```python
from build123d import *

# Parameters (mm, degrees)
SKETCH1_W           = 8
SKETCH1_H           = 8
SKETCH1_R           = 2.5
BOSS_EXTRUDE1_DEPTH = 2
SKETCH5_OUTSIDE_W   = 39.864
SKETCH5_OUTSIDE_H   = 39.864
SKETCH5_OUTSIDE_R   = 4
CUT_EXTRUDE2_DEPTH  = 7.92820323
CUT_EXTRUDE2_DRAFT  = -60


with BuildPart() as part:
    # Sketch1 → Boss-Extrude1 (new, symmetric)
    with BuildSketch(Plane(origin=(0, 0, 0), x_dir=(1, 0, 0), z_dir=(0, 1, 0))):
        Rectangle(SKETCH1_W, SKETCH1_H)
        with Locations(Location((0, 0, 0), (0, 0, 270))):
            Circle(SKETCH1_R, mode=Mode.SUBTRACT)
    extrude(amount=BOSS_EXTRUDE1_DEPTH, both=True)


with BuildPart() as cut_extrude2_tool:
    # Sketch5 outside → Cut-Extrude2 (with draft: the straight prism first)
    with BuildSketch(Plane(origin=(0, 2, 0), x_dir=(1, 0, 0), z_dir=(0, 1, 0))):
        Rectangle(SKETCH5_OUTSIDE_W, SKETCH5_OUTSIDE_H)
        Circle(SKETCH5_OUTSIDE_R, mode=Mode.SUBTRACT)
    extrude(amount=-CUT_EXTRUDE2_DEPTH)
    # Cut-Extrude2: the draft: its side faces are tilted about the plane it starts from
    cut_extrude2_sides = [cut_extrude2_tool.faces().sort_by_distance(p)[0] for p in [
        (0, -1.964101615, 19.932),
        (19.932, -1.964101615, 0),
        (0, -1.964101615, -19.932),
        (-19.932, -1.964101615, 0),
        (-4, -1.964101615, 0),
    ]]
    draft(cut_extrude2_sides, Plane(origin=(0, 2, 0), x_dir=(1, 0, 0), z_dir=(0, 1, 0)), CUT_EXTRUDE2_DRAFT)


with BuildPart() as part_1:
    add(part.part)

    # Cut-Extrude2: cut by cut_extrude2_tool
    add(cut_extrude2_tool.part, mode=Mode.SUBTRACT)


solid = part_1.part
```
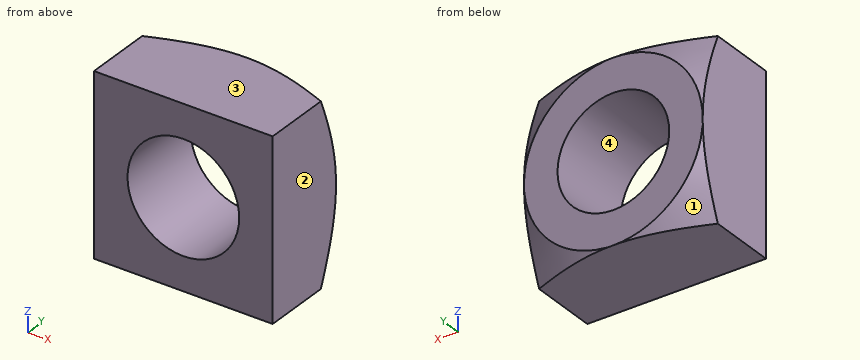
CAD build for the part. Positions are in the model's coordinates, mm. Face numbers are marked on the shaded views. Coordinates: 2 decimals unless noted, no trailing zeros. Order: outer loops, then holes, each group sorted by start corner. A loop starts at its lowest first (then second) coordinate and runs counter-clockwise, first axis right, second up.
(1) Saw through at B-B, the plane y = 1.2. Write the cut outline in (x, z).
Solution:
outline: (-4, -3.61) arc R5.39 ccw to (-3.61, -4) - (3.61, -4) arc R5.39 ccw to (4, -3.61) - (4, 3.61) arc R5.39 ccw to (3.61, 4) - (-3.61, 4) arc R5.39 ccw to (-4, 3.61) - close; hole circle Ø5 at (0, 0)
(2) Saw through at C-C, the plane y = 1.75. Write the cut outline in (x, z).
Solution:
outline: (-4, -1.91) arc R4.43 ccw to (-1.91, -4) - (1.91, -4) arc R4.43 ccw to (4, -1.91) - (4, 1.91) arc R4.43 ccw to (1.91, 4) - (-1.91, 4) arc R4.43 ccw to (-4, 1.91) - close; hole circle Ø5 at (0, 0)
(3) Drill centre lines: L1, parallel to X at y = 0.05, z = 0; L2, parallel to Z at x = -1, y = -0.8; L3, parallel to X at y = -0.35, z = -1.75. Where is each one in solid material? Low to high.
Solution:
L1: x = -4 to -2.5, 2.5 to 4
L2: z = -4 to -2.29, 2.29 to 4
L3: x = -4 to -1.79, 1.79 to 4
(4) Saw through at A-A, the plane y = 0.35. Write the cut outline in (x, z).
Solution:
outline: (-4, -4) - (4, -4) - (4, 4) - (-4, 4) - close; hole circle Ø5 at (0, 0)
(5) Mould opens along X. For the marked faces 1, 2, 3 and 4 say: released by +X, released by -X, zero draft, split by the parting line, or undercut.
Solution:
face 1: released by -X
face 2: released by +X
face 3: zero draft
face 4: undercut
